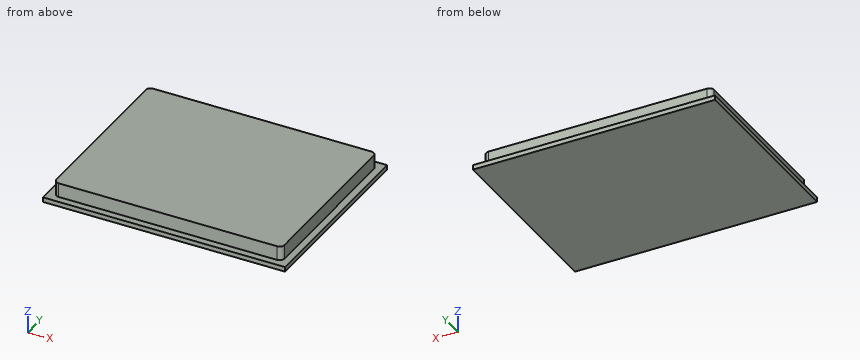
```python
from build123d import *

# Parameters (mm, degrees)
SKETCH_W     = 51
SKETCH_H     = 40
PAD_DEPTH    = 1
PAD001_DEPTH = 3


with BuildPart() as part:
    # Sketch → Pad (new body)
    with BuildSketch(Plane.XY):
        with Locations((-25.5, 20)):
            Rectangle(SKETCH_W, SKETCH_H)
    extrude(amount=PAD_DEPTH)

    # Sketch001 (on DatumPlane) → Pad001 (join)
    with BuildSketch(Plane.XY.offset(1)):
        with BuildLine():
            Line((-48.5, 38.6), (-2.5, 38.6))
            ThreePointArc((-1.5, 37.6), (-1.792893, 38.307107), (-2.5, 38.6))
            Line((-1.5, 37.6), (-1.5, 2.5))
            ThreePointArc((-2.5, 1.5), (-1.792893, 1.792893), (-1.5, 2.5))
            Line((-2.5, 1.5), (-48.5, 1.5))
            ThreePointArc((-49.5, 2.5), (-49.207107, 1.792893), (-48.5, 1.5))
            Line((-49.5, 2.5), (-49.5, 37.6))
            ThreePointArc((-48.5, 38.6), (-49.207107, 38.307107), (-49.5, 37.6))
        make_face()
    extrude(amount=PAD001_DEPTH)


with BuildPart() as part_1:
    # Body placement: moved
    add(part.part.moved(Location((0, 0, -4))))


solid = part_1.part
```
Design review of the part built by this model. Coordinates are the model's own, in mm. Give positions to 0.01 mm unless a question says otherwise; leave off trailing zeros. Write each loop counter-clockwise with the first axis right and the second up, starting at its lowest first coordinate (ties: lowest second). Pieces come first, ordered by that corner, then holes. Notation, with made-up numbers: (-16.75, -34) -> (-6.75, -34) arc R13 cw to (-6.75, -25) -> close; hole circle Ø2 at (63.5, 45). An arc over 180 degrees is marked (long way). Answer in a Markdown table with one row per item.
(1) Clearance check with flat-ended pins moving along their axes: pin 1 (1 mm diameter, centred on x = -22.5, y = 27.5, fed in from +Z); pin 2 (1 mm diameter, centred on x = -39.5, z = -1.5, fed in from -Y). State where each tip first meets the part, or that it passes through.
Results:
| item | result |
|---|---|
| pin 1 | z = 0 |
| pin 2 | y = 1.5 |
(2) Consider section B-B (z = -1.9). State the section outline as (x, y) points, then the cut area to 3 significant figures.
Results:
| item | result |
|---|---|
| outline | (-49.5, 2.5) arc R1 ccw to (-48.5, 1.5) -> (-2.5, 1.5) arc R1 ccw to (-1.5, 2.5) -> (-1.5, 37.6) arc R1 ccw to (-2.5, 38.6) -> (-48.5, 38.6) arc R1 ccw to (-49.5, 37.6) -> close |
| area | 1,780 mm2 |
(3) To check wall thickness, follow probe 1 along X at (y, z) = (34, -2.95); probe 2 along Y at (x, z) = (-26.5, -1.35). State the ranges of each line that lie inside material, in increasing order.
Results:
| item | result |
|---|---|
| probe 1 | -49.5 to -1.5 |
| probe 2 | 1.5 to 38.6 |
(4) Consider section A-A (x = -7). State the section outline as (y, z) points.
Results:
| item | result |
|---|---|
| outline | (0, -4) -> (40, -4) -> (40, -3) -> (38.6, -3) -> (38.6, 0) -> (1.5, 0) -> (1.5, -3) -> (0, -3) -> close |
